from build123d import *

# Parameters (mm, degrees)
F1_DEPTH = 5
F2_R     = 2


with BuildPart() as f1:
    # F0 (on Front) → F1 (new body)
    with BuildSketch(Plane.XZ):
        Polygon((15.221183, 25.589402), (0.426741, 17.017691), (-15.418572, 25.644877), (-29.515327, 16.704283), (-29.515327, -16.961344), (-13.963126, -25.711559), (0.841107, -16.961344), (16.393308, -25.711559), (30.185388, -17.256112), (29.809576, 17.388582), align=None)
        Polygon((-2.354774, -15.121066), (-13.963126, -21.982318), (-13.963126, -8.595468), align=None, mode=Mode.SUBTRACT)
        Polygon((15.221183, 4.428767), (15.221183, 21.288337), (26.722113, 14.817509), (26.722113, -15.223855), (-26.395499, 14.661982), (-15.183636, 21.535588), align=None, mode=Mode.SUBTRACT)
    extrude(amount=F1_DEPTH)

    # F2
    f2_edges = [f1.edges().sort_by_distance(p)[0] for p in [
        (15.221183, -2.5, 25.589402),
        (29.809576, -2.5, 17.388582),
        (30.185388, -2.5, -17.256112),
        (-15.418572, -2.5, 25.644877),
        (16.393308, -2.5, -25.711559),
        (-13.963126, -2.5, -25.711559),
        (-29.515327, -2.5, -16.961344),
        (-29.515327, -2.5, 16.704283),
    ]]
    fillet(f2_edges, radius=F2_R)


solid = f1.part
Geometry: final body of the model. Coordinates: model frame, mm. A direction names the side the tool comes from. Coordinates: 2 decimals unless noted, no trailing zeros. Order: outer loops, then holes, each group sorted by start corner. A loop starts at its lowest first (then second) coordinate and runs counter-clockwise, first axis right, second up.
(1) Section query D-D (z = 0). Return the cut outline in (x, y), plus the area to 3 significant figures.
(2) Section query C-C (x = 7.5). Return the cut outline in (y, z).
(3) Section query B-B (z = 13.5). Return the cut outline in (x, y).
(4) Section query A-A (y = -1.85). Return the cut outline in (x, z), plus the area to 3 significant figures.
(5) First-contact query: pin 1 (1 mm diameter, centred on y = -1.5, z = -12.5, fed in from +X); pin 2 (2 mm diameter, centred on x = 21.5, y = -3.5, fed in from +Z); pin 3 (1.5 mm diameter, centred on y = -1.5, z = 16.5, fed in from +X). Flat tips, straight axial feed; report the tip coordinate or a pass-through.
(6) Access query for faces 1 (the face through (-6.16, -2.46, -21.1)), 2 (the face through (22.6, -2.46, 21.44)), 3 (the face through (-21.8, -2.5, -21.3)), 4 (the face through (-6.875, -2.465, 20.993)), 5 (the face through (26.722, -2, 0)). Directions: +Z, -Z, +X, -X, +Y, -Y. A direction counts if a zero-diameter tool reaches every point of the face in a straight line with its end or side. Return the directions, or none.
(7) Draft query along Z for faces 6 (the face through (-20.87, -2.46, 18.05)), 7 (the face through (-29.515, -2, 0)), 8 (the face through (16.4, -2.54, -25.39)). Return one class per face: pulls with the +Z half, pulls with the -Z half, needs draft (parallel to the pull), parting line crosses it, or undercut.
(8) Material intervals for probe 1 along X at (y, z) = (-0.35, -11); probe 2 along X at (y, z) = (-4.7, 16); probe 3 along Z at (x, y) = (-12, -3.5), sorted ascending.
Solution:
1. outline: (-29.52, -5) - (-0.34, -5) - (-0.34, 0) - (-29.52, 0) - close; (26.72, -5) - (30, -5) - (30, 0) - (26.72, 0) - close
1. area: 162 mm2
2. outline: (-5, -20.71) - (0, -20.71) - (0, -4.41) - (-5, -4.41) - close; (-5, 8.77) - (0, 8.77) - (0, 21.12) - (-5, 21.12) - close
3. outline: (-29.52, -5) - (-24.33, -5) - (-24.33, 0) - (-29.52, 0) - close; (-0.9, -5) - (15.22, -5) - (15.22, 0) - (-0.9, 0) - close; (26.72, -5) - (29.85, -5) - (29.85, 0) - (26.72, 0) - close
4. outline: (-29.52, -15.79) arc R2 ccw to (-28.5, -17.53) - (-14.97, -25.15) arc R2 ccw to (-12.97, -25.12) - (0.84, -16.96) - (15.37, -25.14) arc R2 ccw to (17.4, -25.1) - (29.22, -17.85) arc R2 ccw to (30.17, -16.12) - (29.82, 16.23) arc R2 ccw to (28.8, 17.95) - (16.22, 25.03) arc R2 ccw to (14.23, 25.02) - (0.43, 17.02) - (-14.38, 25.08) arc R2 ccw to (-16.41, 25.01) - (-28.59, 17.29) arc R2 ccw to (-29.52, 15.6) - close; hole (-26.4, 14.66) - (26.72, -15.22) - (26.72, 14.82) - (15.22, 21.29) - (15.22, 4.43) - (-15.18, 21.54) - close; hole (-13.96, -21.98) - (-2.35, -15.12) - (-13.96, -8.6) - close
4. area: 1,640 mm2
5. pin 1: stops at x = 30.14
5. pin 2: stops at z = 22.62
5. pin 3: stops at x = 29.83
6. face 1: -Z, +Y, -Y
6. face 2: +Z, +X, +Y, -Y
6. face 3: -Z, -X, +Y, -Y
6. face 4: +Z, +Y, -Y
6. face 5: +Y, -Y
7. face 6: undercut
7. face 7: needs draft
7. face 8: pulls with the -Z half
8. probe 1: x = -29.52 to -13.96, -9.69 to 19.21, 26.72 to 30.12
8. probe 2: x = -29.48 to -24.21, -5.34 to 15.22, 24.62 to 29.82
8. probe 3: z = -24.55 to -20.82, -9.7 to 6.56, 19.74 to 23.78
